from build123d import *

# Parameters (mm, degrees)
SKETCH1_R           = 12.5
BOSS_EXTRUDE1_DEPTH = 15
SKETCH2_R           = 2
BOSS_EXTRUDE2_DEPTH = 12
FILLET1_R           = 5
FILLET2_R           = 3
CUT_EXTRUDE1_DEPTH  = 5


with BuildPart() as part:
    # Sketch1 → Boss-Extrude1 (new body)
    with BuildSketch(Plane(origin=(0, 0, 0), x_dir=(1, 0, 0), z_dir=(0, 1, 0))):
        with Locations(Location((0, 0, 0), (0, 0, 270))):
            Circle(SKETCH1_R)
    extrude(amount=BOSS_EXTRUDE1_DEPTH)

    # Sketch2 → Boss-Extrude2 (add)
    with BuildSketch(Plane(origin=(0, 15, 0), x_dir=(1, 0, 0), z_dir=(0, 1, 0))):
        with Locations(Location((0, 0, 0), (0, 0, 270))):
            Circle(SKETCH2_R)
    extrude(amount=BOSS_EXTRUDE2_DEPTH)

    # Fillet1
    fillet1_edges = [part.edges().sort_by_distance(p)[0] for p in [
        (0, 15, -12.5),
    ]]
    fillet(fillet1_edges, radius=FILLET1_R)

    # Fillet2
    fillet2_edges = [part.edges().sort_by_distance(p)[0] for p in [
        (0, 0, -12.5),
    ]]
    fillet(fillet2_edges, radius=FILLET2_R)

    # Sketch3 → Cut-Extrude1 (cut)
    with BuildSketch(Plane(origin=(0, 15, 0), x_dir=(1, 0, 0), z_dir=(0, 1, 0))):
        with BuildLine():
            ThreePointArc((3.5, 10.95445115), (0, 11.5), (-3.5, 10.95445115))
            add(Edge.make_bspline(
                [(-3.5, 10.95445115), (0, 2.04554885), (3.5, 10.95445115)],
                knots=[0, 0, 0, 1, 1, 1], degree=2))
        make_face()
        with BuildLine():
            ThreePointArc((10.220840427, 5.271092958), (8.131727984, 8.131727984), (5.271092958, 10.220840427))
            add(Edge.make_bspline(
                [(5.271092958, 10.220840427), (1.446421463, 1.446421463), (10.220840427, 5.271092958)],
                knots=[0, 0, 0, 1, 1, 1], degree=2))
        make_face()
        with BuildLine():
            ThreePointArc((10.95445115, -3.5), (11.5, 0), (10.95445115, 3.5))
            add(Edge.make_bspline(
                [(10.95445115, 3.5), (2.04554885, 0), (10.95445115, -3.5)],
                knots=[0, 0, 0, 1, 1, 1], degree=2))
        make_face()
        with BuildLine():
            ThreePointArc((5.271092958, -10.220840427), (8.131727984, -8.131727984), (10.220840427, -5.271092958))
            add(Edge.make_bspline(
                [(10.220840427, -5.271092958), (1.446421463, -1.446421463), (5.271092958, -10.220840427)],
                knots=[0, 0, 0, 1, 1, 1], degree=2))
        make_face()
        with BuildLine():
            ThreePointArc((-3.5, -10.95445115), (0, -11.5), (3.5, -10.95445115))
            add(Edge.make_bspline(
                [(3.5, -10.95445115), (0, -2.04554885), (-3.5, -10.95445115)],
                knots=[0, 0, 0, 1, 1, 1], degree=2))
        make_face()
        with BuildLine():
            ThreePointArc((-10.220840427, -5.271092958), (-8.131727984, -8.131727984), (-5.271092958, -10.220840427))
            add(Edge.make_bspline(
                [(-5.271092958, -10.220840427), (-1.446421463, -1.446421463), (-10.220840427, -5.271092958)],
                knots=[0, 0, 0, 1, 1, 1], degree=2))
        make_face()
        with BuildLine():
            ThreePointArc((-10.95445115, 3.5), (-11.5, 0), (-10.95445115, -3.5))
            add(Edge.make_bspline(
                [(-10.95445115, -3.5), (-2.04554885, 0), (-10.95445115, 3.5)],
                knots=[0, 0, 0, 1, 1, 1], degree=2))
        make_face()
        with BuildLine():
            ThreePointArc((-5.271092958, 10.220840427), (-8.131727984, 8.131727984), (-10.220840427, 5.271092958))
            add(Edge.make_bspline(
                [(-10.220840427, 5.271092958), (-1.446421463, 1.446421463), (-5.271092958, 10.220840427)],
                knots=[0, 0, 0, 1, 1, 1], degree=2))
        make_face()
    extrude(amount=-CUT_EXTRUDE1_DEPTH, mode=Mode.SUBTRACT)


solid = part.part
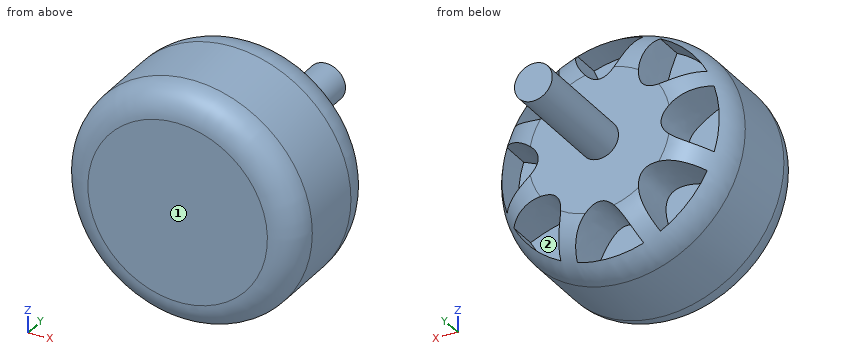
Design review of the part built by this model. Coordinates are the model's own, in mm. Face numbers are marked on the shaded views. A direction names the side the tool comes from. Round coordinates to 2 decimals unless told otherwise and drop trailing zeros. Write each loop counter-clockwise with the first axis right and the second up, starting at its lowest first coordinate (ties: lowest second). Pieces come first, ordered by that corner, then holes. Notation, with made-up numbers: (-16, 56.25) -> (-9, 56.25) arc R18 cw to (-9, 61.25) -> close; hole circle Ø3 at (43, 58). An arc over 180 degrees is marked (long way). One line per item, written item: value. Start each with the question number.
Q1. Add section A-A (y = 23). Give the boundary of the cut face in (x, z).
Q2. To check wall thickness, follow probe 1 along X at (y, z) = (12.25, -5.75); probe 2 along Y at (x, z) = (4.75, -1); probe 3 along X at (y, z) = (12, -10.5). State the ranges of each line that lie inside material, in increasing order.
Q3. Add section B-B (y = 12.5). State how many separate pieces and enclosed holes the cut face has, then the cut area to 3 significant figures.
Q4. Tool access review of the marked faces 1 and 2: name each direction out of +Z, -Z, +X, -X, +Y, -Y from which nothing blocks a thin tool from reaching the whole face with its end or side.
Q5. Insertion check: P1, Ø4, axis at x = 8.5, z = 1.5, coming from the +Y side; P2, Ø4, axis at x = 9.5, z = 9.5, coming from the +Y side; P3, Ø5, axis at x = 3.5, y = 7.5, coming from the +Z side. Each pin has a flat end and moves straight along its axis. Give the tip position at first contact, or say it passes through.
Response:
1. outline: circle Ø4 at (0, 0)
2. probe 1: x = -10.49 to -9.96, -4.12 to 4.12, 9.96 to 10.49
2. probe 2: y = 0 to 15
2. probe 3: x = -5.98 to -3.32, 3.32 to 5.98
3. separate pieces: 1
3. enclosed holes: 8
3. area: 253 mm^2
4. face 1: +Z, -Z, +X, -X, -Y
4. face 2: +Y
5. P1: stops at y = 15
5. P2: stops at y = 13
5. P3: stops at z = 12.46
